Check sheet for the modelled part. Datum: model origin and axes. Units: mm. A direction names the side the tool comes from. Round coordinates to 2 decimals unless told otherwise and drop trailing zeros. Order: outer loops, then holes, each group sorted by start corner. A loop starts at its lowest first (then second) coordinate and runs counter-clockwise, first axis right, second up.
Q1. Scan lines: probe 1 along X at (y, z) = (-37, 22); probe 2 along X at (y, z) = (13.5, 19.5); probe 3 along X at (y, z) = (29, 12.5). Record each from-to range of solid material in increasing order.
Q2. Cross-section at A-A on x = 130. Record the cut outline in (y, z).
Q3. Depth check by flat-ended pin: P1, Ø3, axis at x = 170, y = 40.5, coming from the +Z side. Enter the tip coordinate at first touch or a pass-through.
Q4. Cross-section at C-C on z = 16.5. Record the cut outline in (x, y), then the cut area to 3 significant figures.
Q5. Cross-section at B-B on y = 0. Record the cut outline in (x, z).
Q6. Mould release check, pull along Y, two halves, no side actions. Record for faces 3 (the flat face through (171, 41, 6)), 4 (the flat face through (-3, -80.5, 12)), 5 (the flat face through (225, -1, 12)): +Y half, -Y half, draft (parallel to the pull), parting line (faces both ways), or undercut.
Q7. Set-up check for faces 1 (the flat face through (-3, 1, 0)), 2 (the flat face through (89, -41, 6)): record each of +Z, -Z, +X, -X, +Y, -Y from which the full face is reachable in a straight line by a thin tool's end or side.
from build123d import *

# Parameters (mm, degrees)
SKETCH_1_W          = 450
SKETCH_1_H          = 161
SKETCH_1_R          = 47.5
EXTRUDE_1_DEPTH     = 24
CUT_EXTRUDE_START   = 24
SKETCH_1_3_R        = 5
CUT_EXTRUDE_1_DEPTH = 18


with BuildPart() as part:
    # 草图1 → 凸台-拉伸1 (new body)
    with BuildSketch(Plane.XY):
        Rectangle(SKETCH_1_W, SKETCH_1_H)
        with Locations((130, 0)):
            Circle(SKETCH_1_R, mode=Mode.SUBTRACT)
    extrude(amount=EXTRUDE_1_DEPTH)

    # 草图1<3> → 切除-拉伸1 (cut)
    with BuildSketch(Plane.XY.offset(CUT_EXTRUDE_START)):
        with Locations(Location((89.341360082, 40.658639918, 0), (0, 0, 180))):
            Circle(SKETCH_1_3_R)
        with Locations(Location((170.658639918, 40.658639918, 0), (0, 0, 180))):
            Circle(SKETCH_1_3_R)
        with Locations(Location((170.658639918, -40.658639918, 0), (0, 0, 180))):
            Circle(SKETCH_1_3_R)
        with Locations(Location((89.341360082, -40.658639918, 0), (0, 0, 180))):
            Circle(SKETCH_1_3_R)
    extrude(amount=-CUT_EXTRUDE_1_DEPTH, mode=Mode.SUBTRACT)


solid = part.part
Results found:
1. probe 1: x = -225 to 85.93, 92.75 to 100.21, 159.79 to 167.25, 174.07 to 225
1. probe 2: x = -225 to 84.46, 175.54 to 225
1. probe 3: x = -225 to 92.38, 167.62 to 225
2. outline: (-80.5, 0) - (-47.5, 0) - (-47.5, 24) - (-80.5, 24) - close; (47.5, 0) - (80.5, 0) - (80.5, 24) - (47.5, 24) - close
3. P1: stops at z = 6
4. outline: (-225, -80.5) - (225, -80.5) - (225, 80.5) - (-225, 80.5) - close; hole circle Ø95 at (130, 0); hole circle Ø10 at (89.34, -40.66); hole circle Ø10 at (89.34, 40.66); hole circle Ø10 at (170.66, -40.66); hole circle Ø10 at (170.66, 40.66)
4. area: 65,000 mm2
5. outline: (-225, 0) - (82.5, 0) - (82.5, 24) - (-225, 24) - close; (177.5, 0) - (225, 0) - (225, 24) - (177.5, 24) - close
6. face 3: undercut
6. face 4: -Y half
6. face 5: draft
7. face 1: -Z, +X, -X, +Y, -Y
7. face 2: +Z
